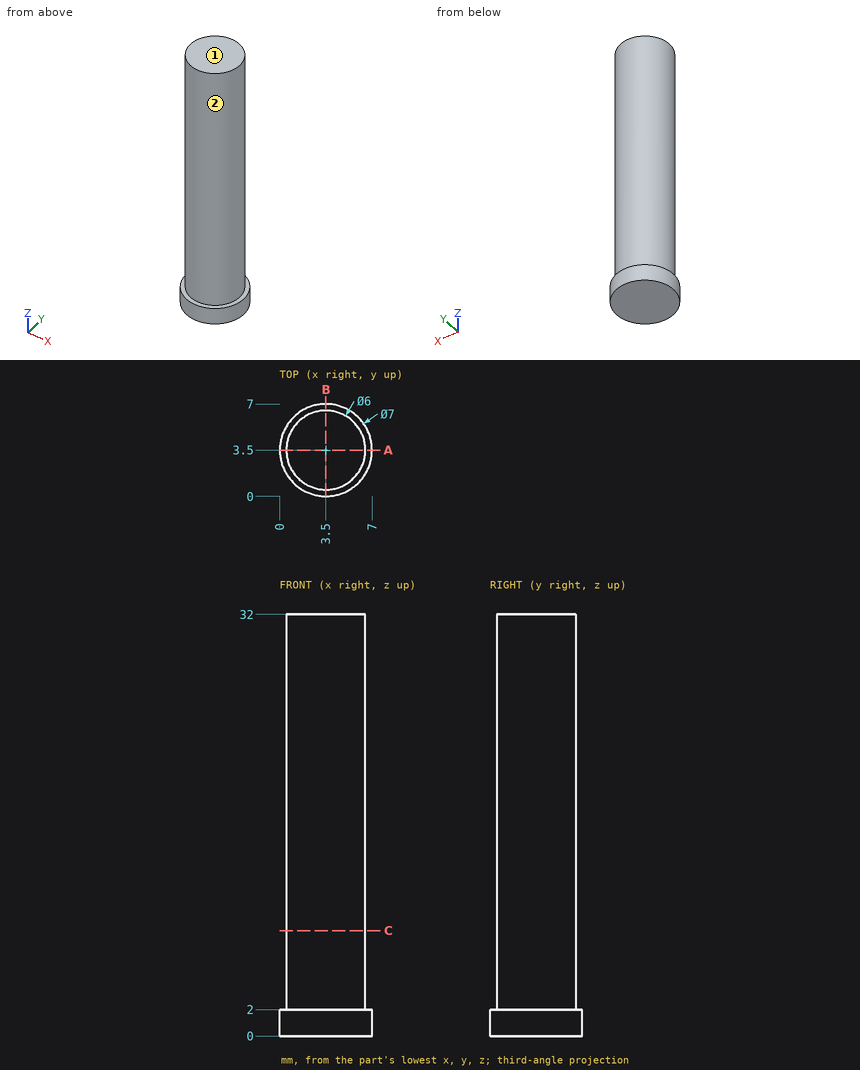
The figure shows three views and two pictorial views of one solid part (mm, origin at its lowest corner). Answer the questions. A direction names the side the tool comes from. Coordinates: 2 decimals unless noted, no trailing zeros. Loops run counter-clockwise (first coordinate to the right, second up) from the corner with the lowest first, then second, coordinate; pieces in that order, holes last. Notation, with made-up numbers: (30.5, 22) - (78.5, 22) arc R18 ccw to (78.5, 55) - close; hole circle Ø1 at (57.25, -39). An arc over 180 degrees is marked (long way). Write item = value, one per line.
1) Each of these flat-tipped pins is pushed along its axis until it touches: P1, Ø1.5, axis at x = 1.5, z = 9, coming from the +Y side; P2, Ø1, axis at y = 4.5, z = 19.5, coming from the +X side; P3, Ø3, axis at y = 3, z = 27.5, coming from the -X side. Where does it stop, or does it pass through?
Responses:
P1 = 6.23
P2 = 6.46
P3 = 0.5
2) Which of the six approach directions +Z, -Z, +X, -X, +Y, -Y give full straight-line access (tool end or side, diameter ignored) to the marked faces 1 and 2?
Responses:
face_1 = +Z, +X, -X, +Y, -Y
face_2 = +Z
3) Section A-A (y = 3.5) is taken. Determine the outline of the cut face in (x, z), plus the area to 3 significant figures.
Responses:
outline = (0, 0) - (7, 0) - (7, 2) - (6.5, 2) - (6.5, 32) - (0.5, 32) - (0.5, 2) - (0, 2) - close
area = 194 mm^2
4) Section C-C (z = 8) is taken. Determine the outline of the cut face in (x, y), plus the area to 3 significant figures.
Responses:
outline = circle Ø6 at (3.5, 3.5)
area = 28.3 mm^2
5) Find the intervals of material crossed by line 1 along Z through (x, y) = (6.75, 3.5); line 2 along Y through (x, z) = (3.5, 10.5); line 3 along X through (y, z) = (1.5, 3), in increasing order.
Responses:
line_1 = 0 to 2
line_2 = 0.5 to 6.5
line_3 = 1.26 to 5.74
